Geometry: final body of the model. Coordinates: model frame, mm. A direction names the side the tool comes from. Give positions to 0.01 mm unless a question says otherwise; leave off trailing zeros. Order: outer loops, then holes, each group sorted by start corner. A loop starts at its lowest first (then second) coordinate and runs counter-clockwise, first axis right, second up. Notation, with made-up numbers: (46.25, 86) -> (105.25, 86) arc R14 cw to (105.25, 108) -> close; hole circle Ø6 at (22, 57.25). An arc over 180 degrees is marked (long way). Answer in a Markdown table with one row per item. Add a question column.
Q1. Pull-direction query (Z, two-part tool) for faces 3 (the face through (-2, -2.4, 0)), 4 (the face through (0.273, 1.266, -17.082)), 5 (the face through (0.273, 1.266, -2.082)), 6 (the face through (0, 0, -20)); classes: +Z half, -Z half, draft (parallel to the pull), parting line (faces both ways), or undercut.
Q2. Cut plane A-A on x = 0. Return the cut outline in (y, z).
Q3. Set-up query: faces 1 (the face through (0.273, 1.266, 12.918)), 2 (the face through (-3, 2.4, 0)). Return all of +Z, -Z, +X, -X, +Y, -Y with unobstructed straight access to the full face (end or side cutting, diameter ignored); none if empty.
Q4. Contact query for a flat-ended pin moving along its axis: P1, Ø4, axis at x = 0, z = 15, coming from the +Y side. Output: stop coordinate, or through.
Q5. Line query: line 1 along Z through (x, y) = (0, 1.4); line 2 along Z through (x, y) = (0, -0.8); line 3 along X through (y, z) = (-1.5, 15). Output: solid intervals per line, ascending. Write a range as from..to.
from build123d import *

# Parameters (mm, degrees)
BOSS_EXTRUDE1_START = 20
BOSS_EXTRUDE1_DEPTH = 40
LPATTERN1_COUNT     = 3
LPATTERN1_PITCH     = 15


with BuildPart() as part:
    # Sketch3 → Boss-Extrude1 (new body)
    with BuildSketch(Plane.XY.offset(BOSS_EXTRUDE1_START)):
        with BuildLine():
            Line((-3.5, -0.074596669), (-3.5, -2))
            Line((-3.5, -2), (-3.1, -2.4))
            Line((-3.1, -2.4), (0.853589838, -2.4))
            ThreePointArc((0.853589838, -2.4), (1.2, -2.2), (1.546410162, -2.4))
            Line((1.546410162, -2.4), (3.1, -2.4))
            Line((3.1, -2.4), (3.5, -2))
            Line((3.5, -2), (3.5, -0.074596669))
            ThreePointArc((3.5, -0.074596669), (3.476025208, 0.006752252), (3.411764706, 0.062096861))
            ThreePointArc((3.411764706, 0.062096861), (3.252980354, 0.161322512), (3.126179073, 0.299089108))
            ThreePointArc((3.126179073, 0.299089108), (3.078284539, 0.343044682), (3.016290807, 0.362608836))
            Line((3.016290807, 0.362608836), (2.586926639, 0.400173333))
            ThreePointArc((2.586926639, 0.400173333), (2.489408399, 0.448264007), (2.45, 0.549602538))
            Line((2.45, 0.549602538), (2.45, 0.850397462))
            ThreePointArc((2.45, 0.850397462), (2.489408399, 0.951735993), (2.586926639, 0.999826667))
            Line((2.586926639, 0.999826667), (3.016290807, 1.037391164))
            ThreePointArc((3.016290807, 1.037391164), (3.078284539, 1.056955318), (3.126179073, 1.100910892))
            ThreePointArc((3.126179073, 1.100910892), (3.252980354, 1.238677488), (3.411764706, 1.337903139))
            ThreePointArc((3.411764706, 1.337903139), (3.476025208, 1.393247748), (3.5, 1.474596669))
            Line((3.5, 1.474596669), (3.5, 2.1))
            Line((3.5, 2.1), (3.2, 2.4))
            Line((3.2, 2.4), (-3.2, 2.4))
            Line((-3.2, 2.4), (-3.5, 2.1))
            Line((-3.5, 2.1), (-3.5, 1.474596669))
            ThreePointArc((-3.5, 1.474596669), (-3.476025208, 1.393247748), (-3.411764706, 1.337903139))
            ThreePointArc((-3.411764706, 1.337903139), (-3.252980354, 1.238677488), (-3.126179073, 1.100910892))
            ThreePointArc((-3.126179073, 1.100910892), (-3.078284539, 1.056955318), (-3.016290807, 1.037391164))
            Line((-3.016290807, 1.037391164), (-2.586926639, 0.999826667))
            ThreePointArc((-2.586926639, 0.999826667), (-2.489408399, 0.951735993), (-2.45, 0.850397462))
            Line((-2.45, 0.850397462), (-2.45, 0.549602538))
            ThreePointArc((-2.45, 0.549602538), (-2.489408399, 0.448264006), (-2.586926639, 0.400173333))
            Line((-2.586926639, 0.400173333), (-3.016290807, 0.362608836))
            ThreePointArc((-3.016290807, 0.362608836), (-3.078284539, 0.343044682), (-3.126179073, 0.299089108))
            ThreePointArc((-3.126179073, 0.299089108), (-3.252980354, 0.161322512), (-3.411764706, 0.062096861))
            ThreePointArc((-3.411764706, 0.062096861), (-3.476025208, 0.006752252), (-3.5, -0.074596669))
        make_face()
    extrude(amount=-BOSS_EXTRUDE1_DEPTH)

    # Sketch4 → Cut-Revolve1 (revolve, cut)
    with BuildSketch(Plane.XY.offset(15)):
        Polygon((0, 2.4), (0, -2.4), (-1.2, -2.4), (-1.2, 0.1), (-2.1, 0.1), (-2.1, 2.4), align=None)
    cut_revolve1 = revolve(axis=Axis((0, 2.4, 15), (0, -1, 0)), mode=Mode.SUBTRACT)

    # LPattern1: Cut-Revolve1 ×3
    with Locations(*[(0, 0, -i * LPATTERN1_PITCH) for i in range(1, LPATTERN1_COUNT)]):
        add(cut_revolve1, mode=Mode.SUBTRACT)


solid = part.part
Completed:
| question | item | result |
|---|---|---|
| 1 | face 3 | draft |
| 1 | face 4 | undercut |
| 1 | face 5 | undercut |
| 1 | face 6 | -Z half |
| 2 | outline | (-2.4, -20) -> (2.4, -20) -> (2.4, -17.1) -> (0.1, -17.1) -> (0.1, -16.2) -> (-2.4, -16.2) -> close; (-2.4, -13.8) -> (0.1, -13.8) -> (0.1, -12.9) -> (2.4, -12.9) -> (2.4, -2.1) -> (0.1, -2.1) -> (0.1, -1.2) -> (-2.4, -1.2) -> close; (-2.4, 1.2) -> (0.1, 1.2) -> (0.1, 2.1) -> (2.4, 2.1) -> (2.4, 12.9) -> (0.1, 12.9) -> (0.1, 13.8) -> (-2.4, 13.8) -> close; (-2.4, 16.2) -> (0.1, 16.2) -> (0.1, 17.1) -> (2.4, 17.1) -> (2.4, 20) -> (-2.4, 20) -> close |
| 3 | face 1 | +Y |
| 3 | face 2 | +Z, -Z, +X, -X, +Y |
| 4 | P1 | stops at y = 0.1 |
| 5 | line 1 | z = -20..-17.1, -12.9..-2.1, 2.1..12.9, 17.1..20 |
| 5 | line 2 | z = -20..-16.2, -13.8..-1.2, 1.2..13.8, 16.2..20 |
| 5 | line 3 | x = -3.5..-1.2, 1.2..3.5 |
